Work out the finished part from the listing and answer in its coordinate system (mm). Face numbers are marked on the shaded views. Give positions to 0.01 mm unless a question says otherwise; leave off trailing zeros. Order: outer loops, then holes, each group sorted by start corner. A loop starts at its lowest first (then second) coordinate and runs counter-clockwise, first axis right, second up.
```python
from build123d import *

# Parameters (mm, degrees)
F0_R     = 9.5
F0_R_2   = 9
F1_DEPTH = 25.4
F0_R_3   = 3.4
F0_R_4   = 2.9
F2_DEPTH = 1
F3_DEPTH = 11.176


with BuildPart() as f1:
    # F0 (on Top) → F1 (new body)
    with BuildSketch(Plane.XY):
        Circle(F0_R)
        Circle(F0_R_2, mode=Mode.SUBTRACT)
    extrude(amount=F1_DEPTH)

    # F0 (on Top) → F2 (join)
    with BuildSketch(Plane.XY):
        Circle(F0_R)
        Circle(F0_R_2, mode=Mode.SUBTRACT)
        Circle(F0_R_2)
        Circle(F0_R_3, mode=Mode.SUBTRACT)
        Circle(F0_R_3)
        Circle(F0_R_4, mode=Mode.SUBTRACT)
        Circle(F0_R_4)
    extrude(amount=-F2_DEPTH)

    # F0 (on Top) → F3 (join)
    with BuildSketch(Plane.XY):
        Circle(F0_R_3)
        Circle(F0_R_4, mode=Mode.SUBTRACT)
    extrude(amount=-F3_DEPTH)


solid = f1.part
```
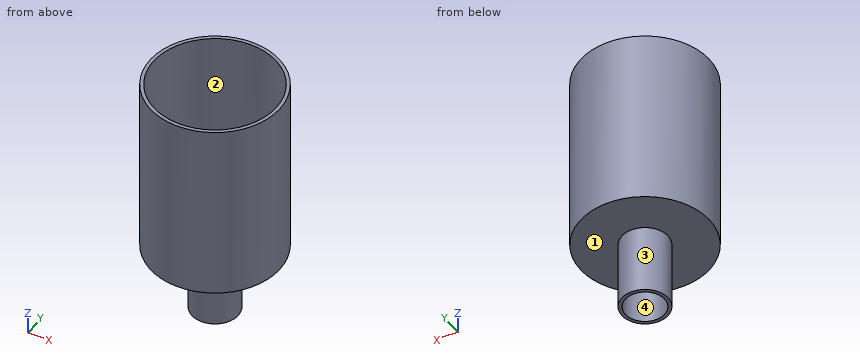
1. The part is cut by section C-C (z = 15.5). Write down the section's boundary in (x, y), then the cut area to 3 significant figures.
Findings below:
outline: circle Ø19 at (0, 0); hole circle Ø18 at (0, 0)
area: 29.1 mm2
2. The part is cut by section A-A (x = 0). Write down the section's boundary in (y, z), then the cut area to 3 significant figures.
Findings below:
outline: (-9.5, -1) - (-3.4, -1) - (-3.4, -11.18) - (-2.9, -11.18) - (-2.9, -1) - (2.9, -1) - (2.9, -11.18) - (3.4, -11.18) - (3.4, -1) - (9.5, -1) - (9.5, 25.4) - (9, 25.4) - (9, 0) - (-9, 0) - (-9, 25.4) - (-9.5, 25.4) - close
area: 54.6 mm2
3. Given P1, Ø8, axis at x = 0, z = -6.5, coming from the -Y side; P2, Ø1.5, axis at x = 1.5, y = 4.5, coming from the +Z side; P3, Ø6, axis at x = -7.5, z = 11, coming from the -Y side, each flat-ended and moving along its own axis, determine where each tip first touches the part or whether it passes through.
Findings below:
P1: stops at y = -3.4
P2: stops at z = 0
P3: stops at y = -8.37
4. The part is cut by section D-D (y = 7). Write down the section's boundary in (x, z), then the cut area to 3 significant figures.
Findings below:
outline: (-6.42, -1) - (6.42, -1) - (6.42, 25.4) - (5.66, 25.4) - (5.66, 0) - (-5.66, 0) - (-5.66, 25.4) - (-6.42, 25.4) - close
area: 51.7 mm2
5. Straight lines are drawn through the part: probe 1 along Y at (x, z) = (0, -5.75); probe 2 along X at (y, z) = (-0.25, 18.5). For each, find the intervals that lie inside material, in ascending order.
Findings below:
probe 1: y = -3.4 to -2.9, 2.9 to 3.4
probe 2: x = -9.5 to -9, 9 to 9.5
6. The mould has two halves that part along Y. Classify the marked faces 1, 2, 3 and 4: pulls with the +Y half, pulls with the -Y half, needs draft (parallel to the pull), parting line crosses it, or undercut.
Findings below:
face 1: needs draft
face 2: undercut
face 3: parting line crosses it
face 4: undercut
